Here's how the part is built. I have some questions about the finished solid (model axes, mm). Face numbers are marked on the shaded views. A direction names the side the tool comes from. Coordinates: 2 decimals unless noted, no trailing zeros. Loops run counter-clockwise (first coordinate to the right, second up) from the corner with the lowest first, then second, coordinate; pieces in that order, holes last. Notation, with made-up numbers: (-28, -28) -> (28, -28) arc R18 ccw to (28, -22) -> close; hole circle Ø2 at (34, 21). An arc over 180 degrees is marked (long way). Answer as a JSON object with one key per item and string values. Group by question number.
1) I want a section at C-C (z = 2.5). Write out the boundary of the cut face in (x, y).
2) Which directions (+Z, -Z, +X, -X, +Y, -Y) give clear straight access to the entire face, cutting with the end or side of a thin tool? Please do the marked faces 4 and 5.
3) I'm going to push flat-ended pins straight in: pin 1 (0.7 mm diameter, centred on y = 2, z = 1.5, fed in from +X); pin 2 (0.7 mm diameter, centred on x = 1.5, y = 1, fed in from -Z); pin 3 (1.5 mm diameter, centred on y = 1, z = -1.5, fed in from +X). Where does each tip first touch, or does it pass through?
4) I want a section at A-A (z = 1.25). Write out the boundary of the cut face in (x, y).
5) I want a section at D-D (x = -2.5). Write out the boundary of the cut face in (y, z), then the cut area to 3 significant figures.
6) If we mould it in two halves opening along X, with no side actions, what happens to the marked faces 1, 2 and 3? For each: +X half, -X half, draft (parallel to the pull), parting line (faces both ways), or undercut.
7) I need wall thicknesses on probe 1 along Z at (x, y) = (-0.75, 2.6); probe 2 along Z at (x, y) = (1, 2.45); probe 3 along X at (y, z) = (2.6, -2). Which ranges of each line are inside material? Lowest first, please. Write a range as [from, to].
8) I want a section at B-B (x = -1.5). Write out the boundary of the cut face in (y, z), then the cut area to 3 significant figures.
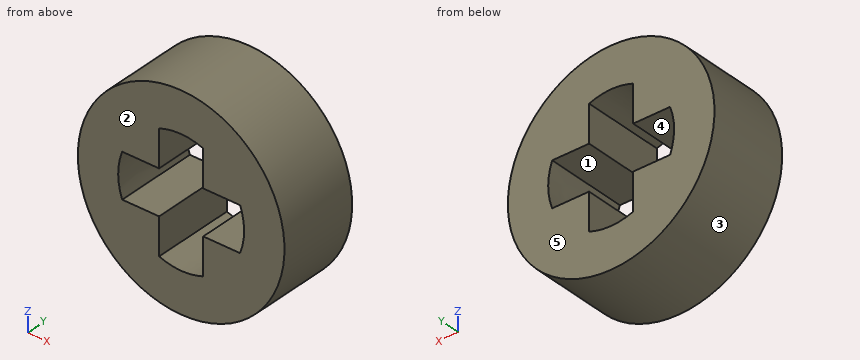
```python
from build123d import *

# Parameters (mm, degrees)
SKETCH1_R           = 3.79
BOSS_EXTRUDE1_DEPTH = 3
CUT_EXTRUDE1_DEPTH  = 3


with BuildPart() as part:
    # Sketch1 → Boss-Extrude1 (new body)
    with BuildSketch(Plane(origin=(0, 0, 0), x_dir=(1, 0, 0), z_dir=(0, 1, 0))):
        with Locations(Location((0, 0, 0), (0, 0, 270))):
            Circle(SKETCH1_R)
    extrude(amount=BOSS_EXTRUDE1_DEPTH)

    # Sketch2 → Cut-Extrude1 (cut)
    with BuildSketch(Plane(origin=(0, 3, 0), x_dir=(1, 0, 0), z_dir=(0, 1, 0))):
        with BuildLine():
            Line((-2.163330765, 0.81), (-0.81, 0.81))
            Line((-0.81, 0.81), (-0.81, 2.163330765))
            add(Edge.make_bspline(
                [(-0.81, 2.163330765), (0, 2.456669235), (0.81, 2.163330765)],
                knots=[0, 0, 0, 1, 1, 1], degree=2))
            Line((0.81, 2.163330765), (0.81, 0.81))
            Line((0.81, 0.81), (2.163330765, 0.81))
            add(Edge.make_bspline(
                [(2.163330765, 0.81), (2.456669235, 0), (2.163330765, -0.81)],
                knots=[0, 0, 0, 1, 1, 1], degree=2))
            Line((2.163330765, -0.81), (0.81, -0.81))
            Line((0.81, -0.81), (0.81, -2.163330765))
            add(Edge.make_bspline(
                [(0.81, -2.163330765), (0, -2.456669235), (-0.81, -2.163330765)],
                knots=[0, 0, 0, 1, 1, 1], degree=2))
            Line((-0.81, -2.163330765), (-0.81, -0.81))
            Line((-0.81, -0.81), (-2.163330765, -0.81))
            add(Edge.make_bspline(
                [(-2.163330765, -0.81), (-2.456669235, 0), (-2.163330765, 0.81)],
                knots=[0, 0, 0, 1, 1, 1], degree=2))
        make_face()
    extrude(amount=-CUT_EXTRUDE1_DEPTH, mode=Mode.SUBTRACT)


solid = part.part
```
Determined:
{
 "1": {"outline": "(-2.85, 0) -> (2.85, 0) -> (2.85, 3) -> (-2.85, 3) -> close"},
 "2": {"face 4": "+Y, -Y", "face 5": "+Z, -Z, +X, -X, +Y"},
 "3": {"pin 1": "x = 3.61", "pin 2": "z = -3.61", "pin 3": "x = 3.72"},
 "4": {"outline": "(-3.58, 0) -> (-0.81, 0) -> (-0.81, 3) -> (-3.58, 3) -> close; (0.81, 0) -> (3.58, 0) -> (3.58, 3) -> (0.81, 3) -> close"},
 "5": {"outline": "(0, -2.85) -> (3, -2.85) -> (3, 2.85) -> (0, 2.85) -> close", "area": "17.1 mm^2"},
 "6": {"face 1": "undercut", "face 2": "draft", "face 3": "parting line"},
 "7": {"probe 1": "[-3.72, -2.18], [2.18, 3.72]", "probe 2": "[-3.66, -0.81], [0.81, 3.66]", "probe 3": "[-3.22, -0.81], [0.81, 3.22]"},
 "8": {"outline": "(0, -3.48) -> (3, -3.48) -> (3, -0.81) -> (0, -0.81) -> close; (0, 0.81) -> (3, 0.81) -> (3, 3.48) -> (0, 3.48) -> close", "area": "16.0 mm^2"}
}
